Autodesk Inventor part; units mm, degrees
ref_plane "YZ Plane" through (0, 0, 0) normal (1, 0, 0) x (0, 1, 0)
ref_plane "XZ Plane" through (0, 0, 0) normal (0, 1, 0) x (-1, 0, 0)
ref_plane "XY Plane" through (0, 0, 0) normal (0, 0, 1) x (1, 0, 0)
sketch "Sketch1" plane through (0, 0, 0) normal (0, 0, 1) x (1, 0, 0)
  circle A0 centre (-0.0139, -12) radius 1.5
  circle A1 centre (-0.0139, 12) radius 1.5
  line L0 (-6.0139, 17.5279) -> (5.9861, 17.5279)
  line L1 (5.9861, 17.5279) -> (5.9861, -17.4721)
  line L2 (5.9861, -17.4721) -> (-6.0139, -17.4721)
  line L3 (-6.0139, -17.4721) -> (-6.0139, 17.5279)
  line L4 (-0.0139, 12) -> (-0.0139, -12)
  line L5 (-0.0139, 12) -> (-0.0139, 5.686)
  ellipse E0 centre (-0.0442, 0.0279) end of major axis (-0.0442, 6.0549) minor radius 4.3359
  point P0 (0, 0)
  point P1 (-0.0139, -12)
  point P2 (-0.0139, 17.5279)
  dimension "d0" = 0
  dimension "d12" = 24
  dimension "d13" = 12
extrude "Extrusion1" add sketch "Sketch1" along normal blind 5
sketch "Sketch2" plane through (0, 0, 5) normal (0, 0, 1) x (1, 0, 0)
  ellipse E0 centre (-0.0442, 0.0279) end of major axis (-0.0442, -5.9992) minor radius 4.3359
  point P0 (0, 0)
extrude "Extrusion2" add sketch "Sketch2" along normal blind 50 and the other way blind 5
chamfer "Chamfer1" distance 2 angle 45 1 edges at (-0.0442, 6.0549, 55)
fillet "Fillet1" radius 1 1 edges at (-0.0139, 17.5279, 5)
fillet "Fillet2" radius 1 1 edges at (-0.0139, -17.4721, 5)
sketch "Sketch3" plane through (0, 0, 5) normal (0, 0, 1) x (1, 0, 0)
  point P0 (0, 0)
sketch "Sketch4" plane through (0, 0, 5) normal (0, 0, 1) x (1, 0, 0)
  point P0 (0, 0)
sketch "Sketch5" plane through (0, 0, 5) normal (0, 0, 1) x (1, 0, 0)
  point P0 (0, 0)
properties part number "apoioM-mod"
Model file for the job. Use its own axes, mm. Give positions to 0.01 mm unless a question says otherwise; leave off trailing zeros. Loops run counter-clockwise (first coordinate to the right, second up) from the corner with the lowest first, then second, coordinate; pieces in that order, holes last. Notation, with made-up numbers: (-10, -4.75) -> (40, -4.75) arc R31 ccw to (40, 26.25) -> close; hole circle Ø11 at (75, -2.5). An arc over 180 degrees is marked (long way). Use a Markdown table: item, result. Add a question column.
(1) Mould opens along X. For faces 1 (the flat face through (-6.014, 0, 2)), 2 (the cylindrical face through (-0.339, 13.464, 2.465)), 3 (the cylindrical face through (-0.339, -10.536, 2.465)), 4 (the flat face through (0, 17.528, 2)) say: +X half, -X half, draft (parallel to the pull), parting line (faces both ways), or undercut.
(2) Drop flat-ended pins along their axis: pin 1 Ø4 at (x, y) = (-0.01, 12) entering from +Z; pin 2 Ø10 at (y, z) = (13.5, 48) entering from -X; pin 3 Ø1.5 at (y, z) = (-4.5, 37.5) entering from -X; pin 4 Ø4 at (x, z) = (3.5, 16) entering from +Y. Give the stop position or say it passes through.
(3) Slice it at B-B on y = 7. List the corners of the cut face in (x, z).
(4) Wall check: line 1 along X through (y, z) = (-12, 2.85); line 2 along Z through (x, y) = (-2.5, 10.5); line 3 along X through (y, z) = (0, 46). Give the ranges that are in metal, low to high.
(5) Slice it at A-A on y = 12. List the corners of the cut face in (x, z).
Filled sheet:
| question | item | result |
|---|---|---|
| 1 | face 1 | -X half |
| 1 | face 2 | undercut |
| 1 | face 3 | undercut |
| 1 | face 4 | draft |
| 2 | pin 1 | z = 5 |
| 2 | pin 2 | through |
| 2 | pin 3 | x = -3.42 |
| 2 | pin 4 | y = 5.66 |
| 3 | outline | (-6.01, 0) -> (5.99, 0) -> (5.99, 5) -> (-6.01, 5) -> close |
| 4 | line 1 | -6.01 to -1.51, 1.49 to 5.99 |
| 4 | line 2 | 0 to 5 |
| 4 | line 3 | -4.38 to 4.29 |
| 5 | outline | (-6.01, 0) -> (-1.51, 0) -> (-1.51, 5) -> (-6.01, 5) -> close; (1.49, 0) -> (5.99, 0) -> (5.99, 5) -> (1.49, 5) -> close |
